Work out the finished part from the listing and answer in its coordinate system (mm). A direction names the side the tool comes from. Give positions to 0.01 mm unless a question says otherwise; leave off trailing zeros. Loops run counter-clockwise (first coordinate to the right, second up) from the corner with the lowest first, then second, coordinate; pieces in that order, holes last.
from build123d import *


with BuildPart() as part:
    # Sketch1 → Revolve1 (revolve)
    with BuildSketch(Plane.XY, mode=Mode.PRIVATE) as revolve1_sk:
        with BuildLine():
            Line((-26.665, 0), (-12.666813836, 160))
            add(Edge.make_bspline(
                [(-12.666813836, 160), (-12.306063793, 164.123391853), (-22.593841128, 176.138404535), (-26.666813836, 170)],
                knots=[0, 0, 0, 0, 1, 1, 1, 1], degree=3))
            add(Edge.make_bspline(
                [(-26.666813836, 170), (-27.754385906, 167.821657289), (-26.181066368, 165.941771752)],
                knots=[0, 0, 0, 1, 1, 1], degree=2))
            Line((-26.181066368, 165.941771752), (-17.959328183, 161.10645018))
            add(Edge.make_bspline(
                [(-17.959328183, 161.10645018), (-15.294831649, 159.923164093), (-15.474513264, 153.742286346), (-20.41748834, 151.432742663), (-23.752458344, 147.815263671), (-20.548654977, 143.94239304), (-19.886137527, 138.797475761), (-19.766435284, 136.001217037), (-19.962779385, 133.756993686)],
                knots=[0, 0, 0, 0, 0.247129658, 0.423699063, 0.532203519, 0.643266944, 0.840064638, 1, 1, 1, 1], degree=3))
            Line((-19.962779385, 133.756993686), (-31.665, 0))
            Line((-31.665, 0), (-26.665, 0))
        make_face()
    revolve(revolve1_sk.sketch.rotate(Axis((0, 0, 0), (0, 1, 0)), 270), axis=Axis((0, 0, 0), (0, 1, 0)))


solid = part.part
Item 1: Flat-ended cylindrical pins translate along their axes: pin 1 Ø6 at (x, y) = (-10.5, 145.5) entering from +Z; pin 2 Ø8 at (x, y) = (-3.5, 69.5) entering from -Z; pin 3 Ø10 at (x, z) = (-4, 14) entering from +Y; pin 4 Ø4 at (x, z) = (8.5, 6) entering from -Y. Find the tip coordinate at first contact, or state that the pin passes through.
Item 2: Find section B-B, the plane y = 36. Write down the section's boundary in (x, z).
Item 3: Consider line 1 (Z direction, x = 8, y = 121); line 2 (Z direction, x = -1, y = 101.5); line 3 (X direction, y = 53, z = -2). Determine where each line is inside the solid, lowest interval first.
Item 4: Find section A-A, the plane y = 75. Write down the section's boundary in (x, z), plus the area to 3 significant figures.
Item 5: Determine the mould class of faces 3 (the face through (21, 0, 17)), 4 (the face through (17.92, 161.34, 3.98)) for opening direction Y: released by +Y, released by -Y, zero draft, split by the parting line, or undercut.
Item 6: For faces 1 (the face through (25.28, 65.94, 5.61)), 2 (the face through (-5.878, 81.12, -18.664)), determine the directions among +Z, -Z, +X, -X, +Y, -Y from which every point of the face is accessible in a straight line to the end or side of a thin tool.
Ans:
1. pin 1: stops at z = 21.33
1. pin 2: stops at z = -25.84
1. pin 3: stops at y = 170.1
1. pin 4: passes through
2. outline: circle Ø57.03 at (0, 0); hole circle Ø47.03 at (0, 0)
3. line 1: z = -19.5 to -13.95, 13.95 to 19.5
3. line 2: z = -22.76 to -17.76, 17.76 to 22.76
3. line 3: x = -26.95 to -21.94, 21.94 to 26.95
4. outline: circle Ø50.21 at (0, 0); hole circle Ø40.21 at (0, 0)
4. area: 710 mm2
5. face 3: released by -Y
5. face 4: undercut
6. face 1: none
6. face 2: -Y
